Design review of the part built by this model. Coordinates are the model's own, in mm. A direction names the side the tool comes from. Coordinates: 2 decimals unless noted, no trailing zeros. Loops run counter-clockwise (first coordinate to the right, second up) from the corner with the lowest first, then second, coordinate; pieces in that order, holes last.
from build123d import *

# Parameters (mm, degrees)
SKETCH1_W           = 43
SKETCH1_H           = 140
SKETCH1_R           = 1.7
SKETCH1_R_2         = 3.5
BOSS_EXTRUDE1_DEPTH = 4
FILLET1_R           = 20
SKETCH2_R           = 1.7
DEPENDANT_DEPTH     = 10


with BuildPart() as part:
    # Sketch1 → Boss-Extrude1 (new body)
    with BuildSketch(Plane.XY):
        with Locations((-1, -50.2)):
            Rectangle(SKETCH1_W, SKETCH1_H)
        with Locations((6.748548523, -12.425907791)):
            Circle(SKETCH1_R, mode=Mode.SUBTRACT)
        with Locations((-8.754354431, -12.425907791)):
            Circle(SKETCH1_R, mode=Mode.SUBTRACT)
        with Locations((-16.505805908, 1)):
            Circle(SKETCH1_R, mode=Mode.SUBTRACT)
        with Locations((-8.754354431, 14.425907791)):
            Circle(SKETCH1_R, mode=Mode.SUBTRACT)
        with Locations((6.748548523, 14.425907791)):
            Circle(SKETCH1_R, mode=Mode.SUBTRACT)
        with Locations((14.5, 1)):
            Circle(SKETCH1_R, mode=Mode.SUBTRACT)
        with Locations((14, -114.2)):
            Circle(SKETCH1_R, mode=Mode.SUBTRACT)
        with Locations((-16, -114.2)):
            Circle(SKETCH1_R, mode=Mode.SUBTRACT)
        with Locations((-1, -103.2)):
            Circle(SKETCH1_R_2, mode=Mode.SUBTRACT)
        with BuildLine():
            Line((6.3, 8), (6.3, -6))
            ThreePointArc((6.3, -6), (-1, -13.3), (-8.3, -6))
            Line((-8.3, -6), (-8.3, 8))
            ThreePointArc((-8.3, 8), (-1, 15.3), (6.3, 8))
        make_face(mode=Mode.SUBTRACT)
        with BuildLine():
            Line((-9, -91.2), (7, -91.2))
            ThreePointArc((7, -91.2), (8.414213562, -90.614213562), (9, -89.2))
            Line((9, -89.2), (9, -81.2))
            ThreePointArc((9, -81.2), (8.414213562, -79.785786438), (7, -79.2))
            Line((7, -79.2), (-9, -79.2))
            ThreePointArc((-9, -79.2), (-10.414213562, -79.785786438), (-11, -81.2))
            Line((-11, -81.2), (-11, -89.2))
            ThreePointArc((-11, -89.2), (-10.414213562, -90.614213562), (-9, -91.2))
        make_face(mode=Mode.SUBTRACT)
    extrude(amount=BOSS_EXTRUDE1_DEPTH)

    # Fillet1
    fillet1_edges = [part.edges().sort_by_distance(p)[0] for p in [
        (-22.5, 19.8, 2),
        (20.5, 19.8, 2),
    ]]
    fillet(fillet1_edges, radius=FILLET1_R)

    # Sketch2 → dependant (cut)
    with BuildSketch(Plane.XY.offset(4)):
        with Locations((-1, -64.401659044)):
            Circle(SKETCH2_R)
        with Locations((6.361215932, -51.651659044)):
            Circle(SKETCH2_R)
        with Locations((-8.361215932, -51.651659044)):
            Circle(SKETCH2_R)
    extrude(amount=-DEPENDANT_DEPTH, mode=Mode.SUBTRACT)


solid = part.part
Q1. Clearance check with flat-ended pins moving along their axes: pin 1 Ø2.5 at (x, y) = (-1, -64.4) entering from +Z; pin 2 Ø8 at (x, y) = (-16.5, -96.5) entering from -Z; pin 3 Ø1.2 at (y, z) = (2, 1.5) entering from -X. State where each tip first meets the part, or that it passes through.
Q2. Take a section at D-D, the plane z = 0.95. Give the number of separate pieces and of enclosed holes in the cut face, then the cut area to 3 significant figures.
Q3. Machinability: for faces 1 (the cylindrical face through (14.486, 14.097, 2.028)), 2 (the flat face through (-8.3, 1, 2)), which of the approach directions +Z, -Z, +X, -X, +Y, -Y give a long, thin tool a straight path to every point of the face, cutting with its end or side? Answer none if there is none.
Q4. The part is to be moulded in two halves that separate along Y. For faces 3 (the flat face through (-1, -120.2, 2)), 4 (the cylindrical face through (-16.797, 13.786, 2.028)), 5 (the cylindrical face through (13.63, -115.86, 1.97)), say which applies: pulls with the +Y half, pulls with the -Y half, needs draft (parallel to the pull), parting line crosses it, or undercut.
Q5. Take a section at B-B, the plane y = -4.5. Write out the cut boundary in (x, z).
Q6. Take a section at A-A, the plane x = -1. Write out the cut boundary in (y, z), then the cut area to 3 significant figures.
Q7. For line 1 (Y direction, x = -1, z = 2.1); line 2 (Y direction, x = 1.5, z = 1.95); line 3 (Y direction, x = -6.5, z = 2.4), list the stretches that pass through material, from the lowest coordinate up.
Q8. Take a section at C-C, the plane y = -114.2. Write out the cut boundary in (x, z).
Entries:
1. pin 1: passes through
1. pin 2: stops at z = 0
1. pin 3: stops at x = -22.44
2. separate pieces: 1
2. enclosed holes: 14
2. area: 5,100 mm2
3. face 1: +Z, -Z, +X, +Y
3. face 2: +Z, -Z
4. face 3: pulls with the -Y half
4. face 4: pulls with the +Y half
4. face 5: undercut
5. outline: (-22.5, 0) - (-8.3, 0) - (-8.3, 4) - (-22.5, 4) - close; (6.3, 0) - (20.5, 0) - (20.5, 4) - (6.3, 4) - close
6. outline: (-120.2, 0) - (-106.7, 0) - (-106.7, 4) - (-120.2, 4) - close; (-99.7, 0) - (-91.2, 0) - (-91.2, 4) - (-99.7, 4) - close; (-79.2, 0) - (-66.1, 0) - (-66.1, 4) - (-79.2, 4) - close; (-62.7, 0) - (-13.3, 0) - (-13.3, 4) - (-62.7, 4) - close; (15.3, 0) - (19.8, 0) - (19.8, 4) - (15.3, 4) - close
6. area: 356 mm2
7. line 1: y = -120.2 to -106.7, -99.7 to -91.2, -79.2 to -66.1, -62.7 to -13.3, 15.3 to 19.8
7. line 2: y = -120.2 to -105.65, -100.75 to -91.2, -79.2 to -12.86, 14.86 to 19.77
7. line 3: y = -120.2 to -91.2, -79.2 to -10.8, 12.8 to 19.4
8. outline: (-22.5, 0) - (-17.7, 0) - (-17.7, 4) - (-22.5, 4) - close; (-14.3, 0) - (12.3, 0) - (12.3, 4) - (-14.3, 4) - close; (15.7, 0) - (20.5, 0) - (20.5, 4) - (15.7, 4) - close
